Could you check a few things on this model? Use its own coordinates, in mm. A direction names the side the tool comes from. Coordinates: 2 decimals unless noted, no trailing zeros. Order: outer loops, then holes, each group sorted by start corner. A loop starts at its lowest first (then second) coordinate and runs counter-clockwise, first axis right, second up. Notation, with made-up numbers: (39, -17.75) -> (58, -17.75) arc R27 ccw to (58, 7.25) -> close; hole circle Ø9 at (69, 58). An arc over 180 degrees is marked (long way). Use a Markdown table: item, result. Add a question column.
1) Which directions (+Z, -Z, +X, -X, +Y, -Y) give clear straight access to the entire face, cutting with the end or side of a thin tool? Please do faces 1 (the cylindrical face through (-14.507, 238.226, 4.077)), 2 (the flat face through (0, 123, -9)).
2) If I drill on L1, parallel to X at y = 20, z = 9.35; L2, parallel to Y at x = 0, z = 9.4; L3, parallel to Y at x = -14.45, z = -3, over which ranges is the centre line in solid material (lowest first)? Write a range as [from, to].
3) Thinking about a two-plate mould opening in Y: for faces 3 (the flat face through (-1.2, 0, 9.6)), 4 (the cylindrical face through (-14.507, 238.226, -3.923)), 5 (the flat face through (0, 123, 9)), which applies, +Y half, -Y half, draft (parallel to the pull), parting line (faces both ways), or undercut?
4) Will this pin go through, and if not, where does the flat tip stop? pin 1 Ø3 at (x, z) = (1.5, 6) entering from +Y.
5) If we section it at A-A (y = 193): Write out the boundary of the cut face in (x, z), plus the area to 3 significant figures.
```python
from build123d import *

# Parameters (mm, degrees)
SKETCH_1_W               = 30
SKETCH_1_H               = 20
SKETCH_1_W_2             = 28
SKETCH_1_H_2             = 18
EXTRUDE_1_DEPTH          = 250
CUT_EXTRUDE_1_DEPTH      = 251.64915719
CUT_EXTRUDE_1_DEPTH_BACK = 251.64915719
SKETCH_2_R               = 1.55
CUT_EXTRUDE_2_DEPTH      = 251.64915719
CUT_EXTRUDE_2_DEPTH_BACK = 251.64915719
SKETCH_3_R               = 2


with BuildPart() as part:
    # 草图1 → 凸台-拉伸1 (new body)
    with BuildSketch(Plane(origin=(0, 0, 0), x_dir=(1, 0, 0), z_dir=(0, 1, 0))):
        Rectangle(SKETCH_1_W, SKETCH_1_H)
        Rectangle(SKETCH_1_W_2, SKETCH_1_H_2, mode=Mode.SUBTRACT)
    extrude(amount=EXTRUDE_1_DEPTH)

    # 草图2 → 切除-拉伸1 (cut, two sides: drawn at the far end of the back side and taken through both)
    with BuildSketch(Plane.XY.offset(-CUT_EXTRUDE_1_DEPTH_BACK)):
        with Locations((0, 28)):
            Circle(SKETCH_2_R)
        with Locations((8, 20)):
            Circle(SKETCH_2_R)
        with Locations((0, 12)):
            Circle(SKETCH_2_R)
        with Locations((-8, 20)):
            Circle(SKETCH_2_R)
    extrude(amount=CUT_EXTRUDE_1_DEPTH + CUT_EXTRUDE_1_DEPTH_BACK, mode=Mode.SUBTRACT)

    # 草图3 → 切除-拉伸2 (cut, two sides: drawn at the far end of the back side and taken through both)
    with BuildSketch(Plane(origin=(0, 0, 0), x_dir=(0, 0, -1), z_dir=(1, 0, 0)).offset(-CUT_EXTRUDE_2_DEPTH_BACK)):
        with Locations((-5, 240)):
            Circle(SKETCH_3_R)
        with Locations((3, 240)):
            Circle(SKETCH_3_R)
    extrude(amount=CUT_EXTRUDE_2_DEPTH + CUT_EXTRUDE_2_DEPTH_BACK, mode=Mode.SUBTRACT)


solid = part.part
```
Answer sheet:
| question | item | result |
|---|---|---|
| 1 | face 1 | +X, -X |
| 1 | face 2 | +Y, -Y |
| 2 | L1 | [-15, -9.55], [-6.45, 6.45], [9.55, 15] |
| 2 | L2 | [0, 10.45], [13.55, 26.45], [29.55, 250] |
| 2 | L3 | [0, 238], [242, 250] |
| 3 | face 3 | -Y half |
| 3 | face 4 | undercut |
| 3 | face 5 | draft |
| 4 | pin 1 | through |
| 5 | outline | (-15, -10) -> (15, -10) -> (15, 10) -> (-15, 10) -> close; hole (-14, -9) -> (14, -9) -> (14, 9) -> (-14, 9) -> close |
| 5 | area | 96.0 mm2 |
